The drawing under review shows one solid part. Ordinate dimensions are in mm from its lowest x, y, z. A direction names the side the tool comes from. Coordinates: 2 decimals unless noted, no trailing zeros. Loops run counter-clockwise (first coordinate to the right, second up) from the corner with the lowest first, then second, coordinate; pieces in that order, holes last. Notation, with made-up numbers: (63.25, -16) - (104.25, -16) arc R17 ccw to (104.25, 7) - close; hole circle Ø4 at (2.5, -25). An arc over 180 degrees is marked (long way). Answer as a JSON object with one key per item and string values. Group by question number.
Item 1: We need section B-B (x = 9). Give the boundary of the cut face in (y, z).
Item 2: Tool access review of the marked faces 1 and 2: name each direction out of +Z, -Z, +X, -X, +Y, -Y from which nothing blocks a thin tool from reaching the whole face with its end or side.
Item 3: To check wall thickness, follow line 1 (Z direction, x = 14, y = 3.5); line 2 (X direction, y = 14, z = 5.5). State the ranges of each line that lie inside material, in increasing order.
Item 4: We need section A-A (y = 3.25). Give the boundary of the cut face in (x, z).
Item 5: Clearance check with flat-ended pins moving along their axes: pin 1 (8 mm diameter, centred on y = 15.5, z = 26.5, fed in from -X); pin 2 (5 mm diameter, centred on x = 10.5, y = 7.5, fed in from -Z). State where each tip first meets the part, or that it passes through.
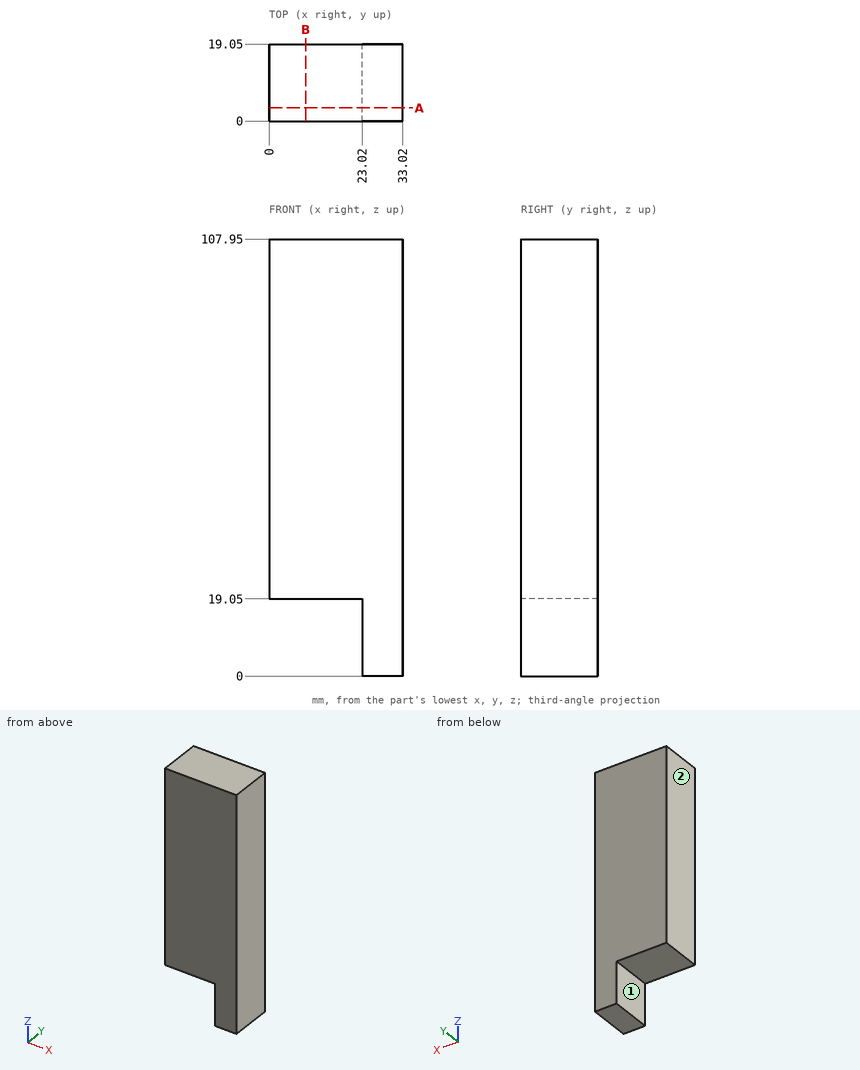
Check sheet entries:
{
 "1": {"outline": "(0, 19.05) - (19.05, 19.05) - (19.05, 107.95) - (0, 107.95) - close"},
 "2": {"face 1": "-Z, -X, +Y, -Y", "face 2": "+Z, -Z, -X, +Y, -Y"},
 "3": {"line 1": "z = 19.05 to 107.95", "line 2": "x = 23.02 to 33.02"},
 "4": {"outline": "(0, 19.05) - (23.02, 19.05) - (23.02, 0) - (33.02, 0) - (33.02, 107.95) - (0, 107.95) - close"},
 "5": {"pin 1": "stops at x = 0", "pin 2": "stops at z = 19.05"}
}
